```python
from build123d import *

# Parameters (mm, degrees)
SKETCH1_W            = 150
SKETCH1_H            = 86
BOSS_EXTRUDE1_DEPTH  = 140
SKETCH2_R            = 1.5
SKETCH2_W            = 78
SKETCH2_H            = 78
SKETCH2_W_2          = 30
SKETCH2_H_2          = 22.5
SKETCH2_W_3          = 21
SKETCH2_H_3          = 15.5
CUT_EXTRUDE1_DEPTH   = 2
SHELL4_START         = 1
SHELL4_OUTLINE_W     = 148
SHELL4_OUTLINE_H     = 84
SHELL4_DEPTH         = 137
SHELL4_START_2       = 138
SHELL4_2_OUTLINE_W   = 148
SHELL4_2_OUTLINE_H   = 84
SHELL4_2_OUTLINE_R   = 2.5
SHELL4_2_OUTLINE_W_2 = 23
SHELL4_2_OUTLINE_H_2 = 17.5
SHELL4_2_OUTLINE_W_3 = 80
SHELL4_2_OUTLINE_H_3 = 80
SHELL4_2_OUTLINE_W_4 = 32
SHELL4_2_OUTLINE_H_4 = 24.5
SHELL4_2_DEPTH       = 1
FILLET1_R            = 10
FILLET2_R            = 5
FILLET3_R            = 2.5


# Read off the part's stored shape, not the designer's step: Shell4
with BuildPart() as part:
    # Sketch1 → Boss-Extrude1 (new body)
    with BuildSketch(Plane(origin=(0, 0, 0), x_dir=(1, 0, 0), z_dir=(0, 1, 0))):
        Rectangle(SKETCH1_W, SKETCH1_H)
    extrude(amount=BOSS_EXTRUDE1_DEPTH)

    # Sketch2 → Cut-Extrude1 (cut)
    with BuildSketch(Plane(origin=(0, 140, 0), x_dir=(1, 0, 0), z_dir=(0, 1, 0))):
        with Locations(Location((69, -37, 0), (0, 0, 270))):
            Circle(SKETCH2_R)
        with Locations(Location((69, 27, 0), (0, 0, 270))):
            Circle(SKETCH2_R)
        with Locations(Location((-69, -37, 0), (0, 0, 270))):
            Circle(SKETCH2_R)
        with Locations(Location((-45, 37, 0), (0, 0, 270))):
            Circle(SKETCH2_R)
        with Locations((23, -0.5)):
            Rectangle(SKETCH2_W, SKETCH2_H)
        with Locations((-45.5, 19.75)):
            Rectangle(SKETCH2_W_2, SKETCH2_H_2)
        with Locations((-45, -15.75)):
            Rectangle(SKETCH2_W_3, SKETCH2_H_3)
    extrude(amount=-CUT_EXTRUDE1_DEPTH, mode=Mode.SUBTRACT)

    # Shell4 outline → Shell4 (cut)
    with BuildSketch(Plane(origin=(0, 0, 0), x_dir=(1, 0, 0), z_dir=(0, 1, 0)).offset(SHELL4_START)):
        Rectangle(SHELL4_OUTLINE_W, SHELL4_OUTLINE_H)
    extrude(amount=SHELL4_DEPTH, mode=Mode.SUBTRACT)

    # Shell4 2 outline → Shell4 2 (cut)
    with BuildSketch(Plane(origin=(0, 0, 0), x_dir=(1, 0, 0), z_dir=(0, 1, 0)).offset(SHELL4_START_2)):
        Rectangle(SHELL4_2_OUTLINE_W, SHELL4_2_OUTLINE_H)
        with Locations((-69, -37)):
            Circle(SHELL4_2_OUTLINE_R, mode=Mode.SUBTRACT)
        with Locations((-45, -15.75)):
            Rectangle(SHELL4_2_OUTLINE_W_2, SHELL4_2_OUTLINE_H_2, mode=Mode.SUBTRACT)
        with Locations((69, -37)):
            Circle(SHELL4_2_OUTLINE_R, mode=Mode.SUBTRACT)
        with Locations((23, -0.5)):
            Rectangle(SHELL4_2_OUTLINE_W_3, SHELL4_2_OUTLINE_H_3, mode=Mode.SUBTRACT)
        with Locations((-45.5, 19.75)):
            Rectangle(SHELL4_2_OUTLINE_W_4, SHELL4_2_OUTLINE_H_4, mode=Mode.SUBTRACT)
        with Locations((-45, 37)):
            Circle(SHELL4_2_OUTLINE_R, mode=Mode.SUBTRACT)
        with Locations((69, 27)):
            Circle(SHELL4_2_OUTLINE_R, mode=Mode.SUBTRACT)
    extrude(amount=SHELL4_2_DEPTH, mode=Mode.SUBTRACT)

    # Fillet1
    fillet1_edges = [part.edges().sort_by_distance(p)[0] for p in [
        (-16, 139, 39.5),
        (-16, 139, -38.5),
        (62, 139, -38.5),
        (62, 139, 39.5),
    ]]
    fillet(fillet1_edges, radius=FILLET1_R)

    # Fillet2
    fillet2_edges = [part.edges().sort_by_distance(p)[0] for p in [
        (-60.5, 139, -8.5),
        (-60.5, 139, -31),
        (-30.5, 139, -31),
        (-30.5, 139, -8.5),
    ]]
    fillet(fillet2_edges, radius=FILLET2_R)

    # Fillet3
    fillet3_edges = [part.edges().sort_by_distance(p)[0] for p in [
        (-55.5, 139, 23.5),
        (-55.5, 139, 8),
        (-34.5, 139, 8),
        (-34.5, 139, 23.5),
    ]]
    fillet(fillet3_edges, radius=FILLET3_R)


solid = part.part
```
Verification items for the finished model (mm, model axes). A direction names the side the tool comes from. Give positions to 0.01 mm unless a question says otherwise; leave off trailing zeros. Order: outer loops, then holes, each group sorted by start corner. A loop starts at its lowest first (then second) coordinate and runs counter-clockwise, first axis right, second up. Notation, with made-up numbers: M -7.5,41.25 L 47.5,41.25 A27 cw 47.5,74.25 Z; hole C -11.5,73 d9. An arc over 180 degrees is marked long. Return JSON: item names as keys, results as strings. Group by question number.
1) Mould release check, pull along X, two halves, no side actions. Record for faces 1 (the face through (75, 69, 1)), 2 (the face through (-1, 69, -43)), 3 (the face through (-1, 1, -1)): pulls with the +X half, pulls with the -X half, needs draft (parallel to the pull), parting line crosses it, or undercut.
2) Scan lines: line 1 (Z direction, x = 69, y = 139.25); line 2 (Z direction, x = 51.5, y = 7); line 3 (Z direction, x = 69, y = 138.45). Record each from-to range of solid material in increasing order.
3) Section check D-D on x = 29.5. Record the cut outline in (y, z).
4) Section check A-A on y = 29.5. Record the cut outline in (x, z), and give its area (3 significant figures).
5) Section check C-C on x = -51. Record the cut outline in (y, z).
6) Access from +Z, -Z, +X, -X, +Y, -Y to the whole of each face (thin tool, end or side, straight path). Record for faces 4 (the face through (-18, 140, -1)), 5 (the face through (-13.15, 138.99, 36.49)), 6 (the face through (-45.1, 138, 7.3)).
7) Section check B-B on x = -19.5. Record the cut outline in (y, z), and give its area (3 significant figures).
8) Go/stop test with flat-tipped pins: pin 1 Ø5 at (x, z) = (-14, 14) entering from -Y; pin 2 Ø3 at (x, z) = (57.5, -20.5) entering from +Y. Record where each tip stops, or that it passes through.
Answer block:
{
 "1": {"face 1": "pulls with the +X half", "face 2": "needs draft", "face 3": "undercut"},
 "2": {"line 1": "z = -43 to -28.5, -25.5 to 35.5, 38.5 to 43", "line 2": "z = -43 to -42, 42 to 43", "line 3": "z = -43 to -42, -29.5 to -28.5, -25.5 to -24.5, 34.5 to 35.5, 38.5 to 39.5, 42 to 43"},
 "3": {"outline": "M 0,-43 L 140,-43 L 140,-38.5 L 138,-38.5 L 138,-39.5 L 139,-39.5 L 139,-42 L 1,-42 L 1,42 L 139,42 L 139,40.5 L 138,40.5 L 138,39.5 L 140,39.5 L 140,43 L 0,43 Z"},
 "4": {"outline": "M -75,-43 L 75,-43 L 75,43 L -75,43 Z; hole M -74,-42 L 74,-42 L 74,42 L -74,42 Z", "area": "468 mm^2"},
 "5": {"outline": "M 0,-43 L 140,-43 L 140,-31 L 138,-31 L 138,-32 L 139,-32 L 139,-42 L 1,-42 L 1,42 L 139,42 L 139,24.5 L 138,24.5 L 138,23.5 L 140,23.5 L 140,43 L 0,43 Z; M 138,-8.5 L 140,-8.5 L 140,8 L 138,8 L 138,7 L 139,7 L 139,-7.5 L 138,-7.5 Z"},
 "6": {"face 4": "+Z, -Z, +X, -X, +Y", "face 5": "+Y", "face 6": "none"},
 "7": {"outline": "M 0,-43 L 140,-43 L 140,43 L 0,43 Z; hole M 1,-42 L 139,-42 L 139,42 L 1,42 Z", "area": "448 mm^2"},
 "8": {"pin 1": "stops at y = 0", "pin 2": "stops at y = 1"}
}
